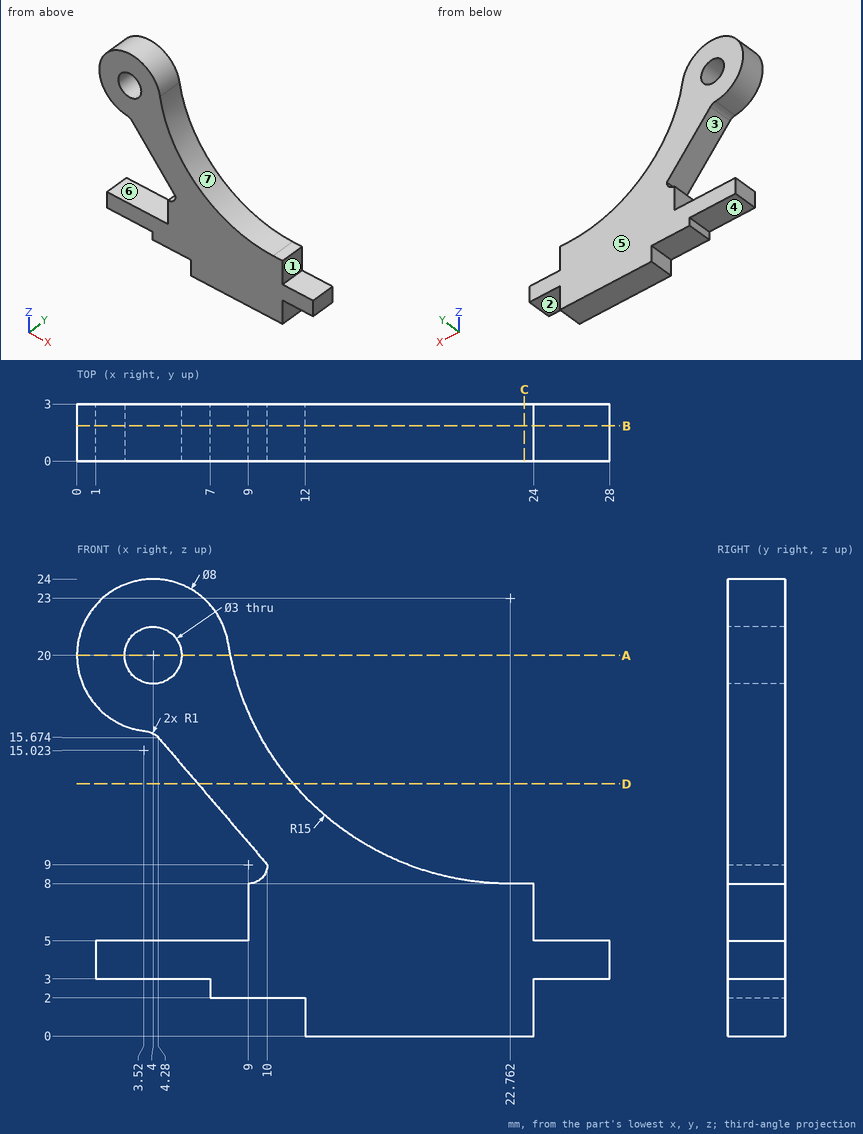
The drawing under review shows one solid part. Ordinate dimensions are in mm from its lowest x, y, z. A direction names the side the tool comes from. Round coordinates to 2 decimals unless told otherwise and drop trailing zeros. Write each loop counter-clockwise with the first axis right and the second up, starting at its lowest first coordinate (ties: lowest second). Pieces come first, ordered by that corner, then holes.
(1) Mouldability with a two-part tool opening along Z and no side actions: class the marked faces 5, 6 and 7 as +Z half, -Z half, draft (parallel to the pull), parting line (faces both ways), or undercut.
(2) We need section A-A on z = 20. Give the boundary of the cut face in (x, y) (1 decimal), and give its area (3 significant figures).
(3) We need section B-B on y = 1.85. Give the boundary of the cut face in (x, z), and give its area (3 significant figures).
(4) We need section D-D on z = 13.25. Give the boundary of the cut face in (x, y), and give its area (3 significant figures).
(5) Machinability: for the marked faces 1, 2, 3 and 4, which of the approach directions +Z, -Z, +X, -X, +Y, -Y give a long, thin tool a straight path to every point of the face, cutting with its end or side? Answer none if there is none.
(6) Wall thickness on L1, parallel to Z at x = 2.75, y = 1.6; L2, parallel to Z at x = 4, y = 1; L3, parallel to Z at x = 24.5, y = 2.65: over which ranges is each line inside the solid? List them lowest first.
(7) Insertion check: pin 1 (1.5 mm diameter, centred on y = 1, z = 16.5, fed in from +X); pin 2 (1.6 mm diameter, centred on y = 1.5, z = 0.5, fed in from -X); pin 3 (1.5 mm diameter, centred on x = 25, y = 1, fed in from +Z). Each pin has a flat end and moves straight along its axis. Give the tip position at first contact, or say it passes through.
(8) We need section C-C on x = 23.5. Give the boundary of the cut face in (y, z), and give its area (3 significant figures).
Findings below:
1. face 5: draft
1. face 6: undercut
1. face 7: +Z half
2. outline: (0, 0) - (2.5, 0) - (2.5, 3) - (0, 3) - close; (5.5, 0) - (8.1, 0) - (8.1, 3) - (5.5, 3) - close
2. area: 15.2 mm2
3. outline: (1, 3) - (7, 3) - (7, 2) - (12, 2) - (12, 0) - (24, 0) - (24, 3) - (28, 3) - (28, 5) - (24, 5) - (24, 8) - (22.76, 8) arc R15 cw to (7.95, 20.63) arc R4 ccw (long way) to (3.62, 16.02) arc R1 cw to (4.28, 15.67) - (10, 9) arc R1 cw to (9, 8) - (9, 5) - (1, 5) - close; hole circle Ø3 at (4, 20)
3. area: 237 mm2
4. outline: (6.36, 0) - (11.36, 0) - (11.36, 3) - (6.36, 3) - close
4. area: 15.0 mm2
5. face 1: +Z, +X, +Y, -Y
5. face 2: -Z, +X, +Y, -Y
5. face 3: -X, +Y, -Y
5. face 4: -Z, -X, +Y, -Y
6. L1: z = 3 to 5, 16.2 to 19.17, 20.83 to 23.8
6. L2: z = 3 to 5, 15.9 to 18.5, 21.5 to 24
6. L3: z = 3 to 5
7. pin 1: stops at x = 9.63
7. pin 2: stops at x = 12
7. pin 3: stops at z = 5
8. outline: (0, 0) - (3, 0) - (3, 8) - (0, 8) - close
8. area: 24.0 mm2
